Could you check a few things on this model? Use its own coordinates, in mm. A direction names the side the tool comes from. Coordinates: 2 decimals unless noted, no trailing zeros. Order: outer loops, then holes, each group sorted by start corner. A loop starts at its lowest first (then second) coordinate and runs counter-clockwise, first axis right, second up. Notation, with made-up numbers: (-6, 68) - (29, 68) arc R16 cw to (29, 81) - close; hole circle Ø10 at (16, 83). An arc over 180 degrees is marked (long way). Answer as a JSON object with one key per item and string values. Group by question number.
(1) Imagine slicing it at A-A, the plane x = 0. Write out the boundary of the cut face in (y, z) (3 decimals).
(2) Imagine slicing it at D-D, the plane x = 5.25. Write out the boundary of the cut face in (y, z), and give its area (3 significant figures).
(3) We'd pull the mould along X, two halves only. Please class faces 1 (the flat face through (0, -35, -1.6)), 2 (the flat face through (-9.195, -28, 12)), 3 (the cylindrical face through (-7.956, 7.296, 3.131)): pulls with the +X half, pulls with the -X half, needs draft (parallel to the pull), parting line crosses it, or undercut.
(4) Will these pins go through, and if not, where does the flat tip stop? P1, Ø6.5, axis at y = -26.797, z = 15.875, coming from the -X side; P2, Ø12, axis at x = 4, y = -12, coming from the +Z side; P3, Ø6, axis at x = 10, z = 7, coming from the -Y side; P4, Ø6, axis at x = -0.5, y = -29, coming from the -Z side.
(5) Please list where these lines run through material, in increasing order: probe 1 along Y at (x, z) = (0, 3.25) (3 decimals); probe 2 along Z at (x, y) = (5.25, 11); probe 3 along X at (y, z) = (-30.5, 7.5).
(6) Imagine slicing it at C-C, the plane y = 3. Write out the boundary of the cut face in (x, z).
(7) Which directions (+Z, -Z, +X, -X, +Y, -Y) give clear straight access to the entire face, cutting with the end or side of a thin tool? Please do faces 4 (the flat face through (-12, -17.272, 13)), 5 (the flat face through (0, -16, 6.35)), 6 (the cylindrical face through (-11.62, -23.8, 17.79)), 7 (the flat face through (13.97, -18, 3)), 8 (the flat face through (0, -14, 0)).
(8) Imagine slicing it at B-B, the plane z = 14. Write out the boundary of the cut face in (x, y), and give its area (3 significant figures).
from build123d import *

# Parameters (mm, degrees)
SKETCH2_R           = 10.795
BOSS_EXTRUDE1_DEPTH = 6.35
SKETCH4_W           = 27.94
SKETCH4_H           = 3.175
BOSS_EXTRUDE2_DEPTH = 7.9502
SKETCH5_R           = 3.556
BOSS_EXTRUDE3_DEPTH = 4.7752
FILLET2_R           = 3.175


with BuildPart() as part:
    # Sketch2 → Boss-Extrude1 (new body)
    with BuildSketch(Plane.XY):
        with BuildLine():
            Line((-13.97, 0), (-13.97, -33.147))
            Line((-13.97, -33.147), (13.97, -33.147))
            Line((13.97, -33.147), (13.97, 0))
            ThreePointArc((13.97, 0), (0, 13.97), (-13.97, 0))
        make_face()
        Circle(SKETCH2_R, mode=Mode.SUBTRACT)
    extrude(amount=BOSS_EXTRUDE1_DEPTH)

    # Sketch4 → Boss-Extrude2 (add)
    with BuildSketch(Plane.XY.offset(6.35)):
        with Locations((0, -34.7345)):
            Rectangle(SKETCH4_W, SKETCH4_H)
    extrude(amount=-BOSS_EXTRUDE2_DEPTH)

    # Sketch5 → Boss-Extrude3 (add)
    with BuildSketch(Plane.ZY.offset(13.97)):
        with BuildLine():
            Line((6.35, -36.322), (15.875, -36.322))
            ThreePointArc((15.875, -36.322), (25.4, -26.797), (15.875, -17.272))
            Line((15.875, -17.272), (6.35, -17.272))
            Line((6.35, -17.272), (6.35, -36.322))
        make_face()
        with Locations((15.875, -26.797)):
            Circle(SKETCH5_R, mode=Mode.SUBTRACT)
    extrude(amount=-BOSS_EXTRUDE3_DEPTH)

    # Fillet2
    fillet2_edges = [part.edges().sort_by_distance(p)[0] for p in [
        (-11.5824, -17.272, 6.35),
    ]]
    fillet(fillet2_edges, radius=FILLET2_R)


solid = part.part
Result set:
{
 "1": {"outline": "(-36.322, -1.6) - (-33.147, -1.6) - (-33.147, 0) - (-10.795, 0) - (-10.795, 6.35) - (-36.322, 6.35) - close; (10.795, 0) - (13.97, 0) - (13.97, 6.35) - (10.795, 6.35) - close"},
 "2": {"outline": "(-36.32, -1.6) - (-33.15, -1.6) - (-33.15, 0) - (-9.43, 0) - (-9.43, 6.35) - (-36.32, 6.35) - close; (9.43, 0) - (12.95, 0) - (12.95, 6.35) - (9.43, 6.35) - close", "area": "198 mm^2"},
 "3": {"face 1": "needs draft", "face 2": "pulls with the +X half", "face 3": "undercut"},
 "4": {"P1": "passes through", "P2": "stops at z = 6.35", "P3": "stops at y = -36.32", "P4": "stops at z = 0"},
 "5": {"probe 1": "y = -36.322 to -10.795, 10.795 to 13.97", "probe 2": "z = 0 to 6.35", "probe 3": "x = -13.97 to -9.19"},
 "6": {"outline": "(-13.64, 0) - (-10.37, 0) - (-10.37, 6.35) - (-13.64, 6.35) - close; (10.37, 0) - (13.64, 0) - (13.64, 6.35) - (10.37, 6.35) - close"},
 "7": {"face 4": "+Z, +X, -X, +Y", "face 5": "+Z, +X, +Y", "face 6": "+X, -X", "face 7": "+Z, -Z, +X, +Y, -Y", "face 8": "-Z, +X, -X, +Y"},
 "8": {"outline": "(-13.97, -36.32) - (-9.19, -36.32) - (-9.19, -29.82) - (-13.97, -29.82) - close; (-13.97, -23.78) - (-9.19, -23.78) - (-9.19, -17.27) - (-13.97, -17.27) - close", "area": "62.1 mm^2"}
}
